Study the drawing (mm; zero at the part's minimum x, y, z) and answer. Round coordinates to 2 decimals unless told otherwise and drop trailing zeros. Write each loop counter-clockwise with the first axis right and the second up, starting at its lowest first coordinate (ties: lowest second). Pieces come first, ordered by that corner, then holes. Notation, with made-up numbers: (68.5, 18.5) -> (75.5, 18.5) arc R21 cw to (75.5, 39.5) -> close; hole circle Ø4 at (1, 9). An arc over 180 degrees is marked (long way). Return JSON: item names as keys, results as strings.
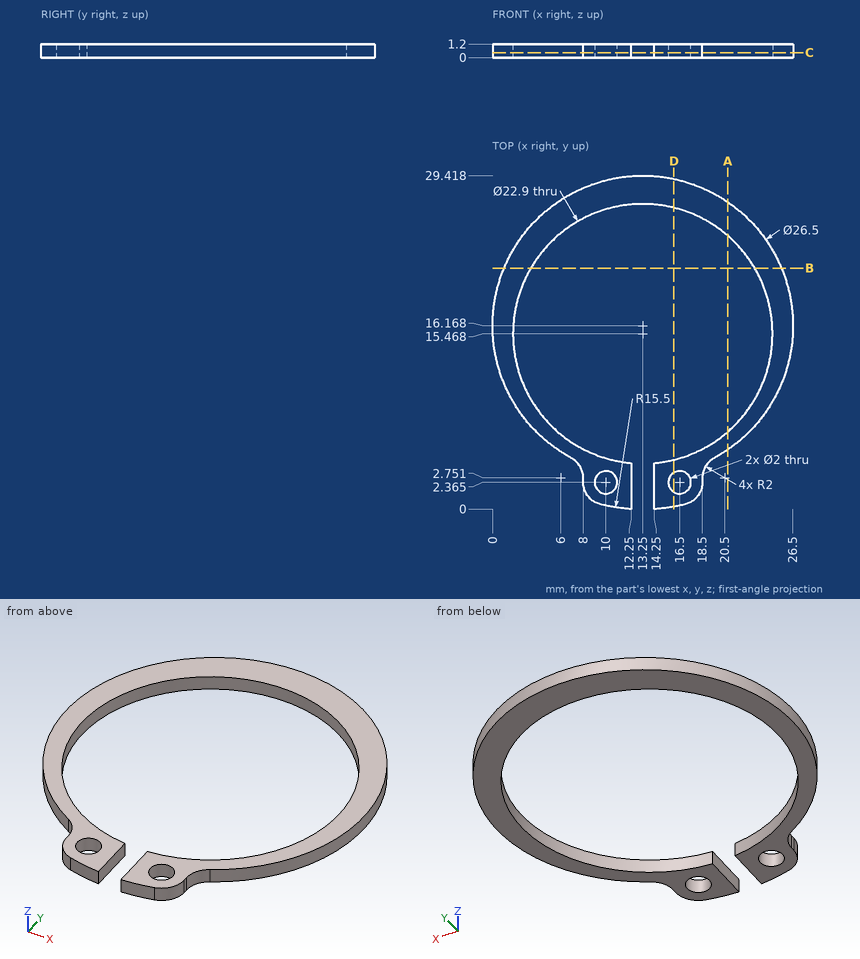
Item 1: Section C-C (z = 0.45) is taken. State how many separate pieces and enclosed holes the cut face has.
Worked answers:
{"separate pieces": "1", "enclosed holes": "2"}
Item 2: Section D-D (x = 16) is taken. Give the vertices of the cut face in (y, z).
Worked answers:
{"outline": "(0.21, 0) -> (1.5, 0) -> (1.5, 1.2) -> (0.21, 1.2) -> close; (3.23, 0) -> (4.35, 0) -> (4.35, 1.2) -> (3.23, 1.2) -> close; (26.58, 0) -> (29.13, 0) -> (29.13, 1.2) -> (26.58, 1.2) -> close"}
Item 3: Section A-A (x = 20.75) is taken. Give the vertices of the cut face in (y, z) (1 decimal).
Worked answers:
{"outline": "(5.2, 0) -> (6.8, 0) -> (6.8, 1.2) -> (5.2, 1.2) -> close; (24.1, 0) -> (27.1, 0) -> (27.1, 1.2) -> (24.1, 1.2) -> close"}
Item 4: A flat-ended cylindrical pin translates along its axis: pin 1 (1.8 mm diameter, centred on x = 10, y = 2.36, fed in from -Z). Find the tip coordinate at first contact, or state that the pin passes through.
Worked answers:
{"pin 1": "passes through"}
Item 5: Section B-B (y = 21.25) is taken. Give the vertices of the cut face in (x, z).
Worked answers:
{"outline": "(1.01, 0) -> (3.37, 0) -> (3.37, 1.2) -> (1.01, 1.2) -> close; (23.13, 0) -> (25.49, 0) -> (25.49, 1.2) -> (23.13, 1.2) -> close"}
Item 6: Straight lines are drawn through the part: L1, parallel to Y at x = 16.5, z = 0.1 (1 decimal); L2, parallel to X at y = 2, z = 1.1; L3, parallel to Y at x = 3.5, z = 1.05 (1 decimal). For each, find the intervals that lie inside material, in ascending order. Write a range as [from, to].
Worked answers:
{"L1": "y = [0.3, 1.4], [3.4, 4.5], [26.4, 29]", "L2": "x = [8.03, 9.07], [10.93, 12.25], [14.25, 15.57], [17.43, 18.47]", "L3": "y = [7.2, 9.5], [21.5, 25.1]"}
